from build123d import *

# Parameters (mm, degrees)
SKETCH1_R           = 21.5
SKETCH1_R_2         = 3.935
BOSS_EXTRUDE1_DEPTH = 6
SKETCH2_R           = 21.5
SKETCH2_R_2         = 2.146170777
BOSS_EXTRUDE2_DEPTH = 2
SKETCH3_W           = 47.979392496
SKETCH3_H           = 15
CUT_EXTRUDE1_DEPTH  = 1


with BuildPart() as part:
    # Sketch1 → Boss-Extrude1 (new body)
    with BuildSketch(Plane(origin=(0, 0, 0), x_dir=(1, 0, 0), z_dir=(0, 1, 0))):
        with Locations(Location((0, 0, 0), (0, 0, 270))):  # turned: the seam where the file's is
            Circle(SKETCH1_R)
        with Locations(Location((0, 0, 0), (0, 0, 270))):  # turned: the seam where the file's is
            Circle(SKETCH1_R_2, mode=Mode.SUBTRACT)
    extrude(amount=BOSS_EXTRUDE1_DEPTH)

    # Sketch2 → Boss-Extrude2 (add)
    with BuildSketch(Plane(origin=(0, 6, 0), x_dir=(1, 0, 0), z_dir=(0, 1, 0))):
        with Locations(Location((0, 0, 0), (0, 0, 270))):  # turned: the seam where the file's is
            Circle(SKETCH2_R)
        with Locations(Location((0, 0, 0), (0, 0, 270))):  # turned: the seam where the file's is
            Circle(SKETCH2_R_2, mode=Mode.SUBTRACT)
    extrude(amount=BOSS_EXTRUDE2_DEPTH)

    # Sketch3 → Cut-Extrude1 (cut)
    with BuildSketch(Plane(origin=(0, 8, 0), x_dir=(1, 0, 0), z_dir=(0, 1, 0))):
        Rectangle(SKETCH3_W, SKETCH3_H)
    extrude(amount=-CUT_EXTRUDE1_DEPTH, mode=Mode.SUBTRACT)


solid = part.part
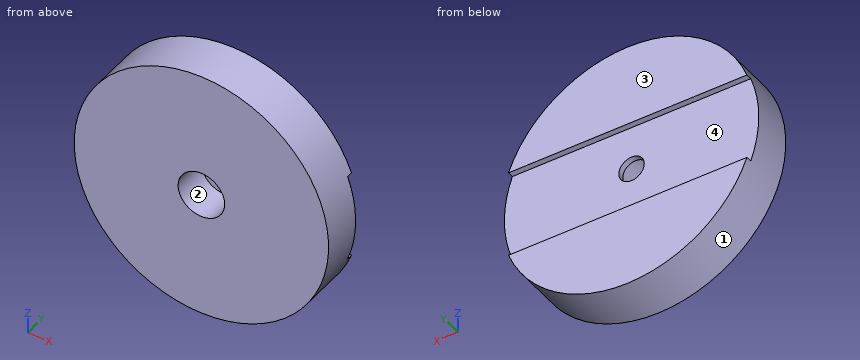
Model file for the job. Use its own axes, mm. Face numbers are marked on the shaded views. Round coordinates to 2 decimals unless told otherwise and drop trailing zeros. Loops run counter-clockwise (first coordinate to the right, second up) from the corner with the lowest first, then second, coordinate; pieces in that order, holes last. Notation, with made-up numbers: (-1.75, 40) -> (7.25, 40) arc R23 ccw to (7.25, 64) -> close; hole circle Ø8 at (22.25, -37.75). An arc over 180 degrees is marked (long way). Answer as CSV lines item,"result". Start each with the question number.
1) Pin check, flat tips, straight feed: P1, Ø4.5, axis at x = 5, z = -1.5, coming from the +Y side; P2, Ø3, axis at x = 4.5, y = 5, coming from the +Z side; P3, Ø0.5, axis at x = -7, y = 7.5, coming from the +Z side. Stop position of each tip, or through.
2) Slice it at B-B (x = 0). List the corners of the cut face in (y, z) (3 decimals).
3) Slice it at D-D (y = 0.75). List the corners of the cut face in (x, z) (3 decimals), plus the area to 3 significant figures.
4) Slice it at A-A (z = 0). List the corners of the cut face in (x, y) (3 decimals).
5) Probe line 1 along X through (y, z) = (4.75, 0) (3 decimals); line 2 along Z through (x, y) = (0, 6.25). List the from-to ranges inside material, lowest first.
6) Mould opens along Z. For the marked faces 1, 2, 3 and 4 say: +Z half, -Z half, draft (parallel to the pull), parting line (faces both ways), or undercut.
7) Slice it at C-C (x = 4.5). List the corners of the cut face in (y, z).
Filled in:
1,P1,"stops at y = 7"
1,P2,"stops at z = 21.29"
1,P3,"stops at z = 20.41"
2,outline,"(0, -21.5) -> (8, -21.5) -> (8, -7.5) -> (7, -7.5) -> (7, -2.146) -> (6, -2.146) -> (6, -3.935) -> (0, -3.935) -> close; (0, 3.935) -> (6, 3.935) -> (6, 2.146) -> (7, 2.146) -> (7, 7.5) -> (8, 7.5) -> (8, 21.5) -> (0, 21.5) -> close"
3,outline,"circle Ø43 at (0, 0); hole circle Ø7.87 at (0, 0)"
3,area,"1,400 mm2"
4,outline,"(-21.5, 0) -> (-3.935, 0) -> (-3.935, 6) -> (-2.146, 6) -> (-2.146, 7) -> (-21.5, 7) -> close; (2.146, 6) -> (3.935, 6) -> (3.935, 0) -> (21.5, 0) -> (21.5, 7) -> (2.146, 7) -> close"
5,line 1,"x = -21.5 to -3.935, 3.935 to 21.5"
5,line 2,"z = -21.5 to -2.15, 2.15 to 21.5"
6,face 1,"parting line"
6,face 2,"undercut"
6,face 3,"draft"
6,face 4,"undercut"
7,outline,"(0, -21.02) -> (8, -21.02) -> (8, -7.5) -> (7, -7.5) -> (7, 7.5) -> (8, 7.5) -> (8, 21.02) -> (0, 21.02) -> close"
